Geometry: see drawing. Coordinates: mm, zero at the bounding-box minimum. A direction names the side the tool comes from. Coordinates: 2 decimals unless noted, no trailing zeros. Order: outer loops, then holes, each group sorted by start corner. A loop starts at its lowest first (then second) coordinate and runs counter-clockwise, first axis right, second up.
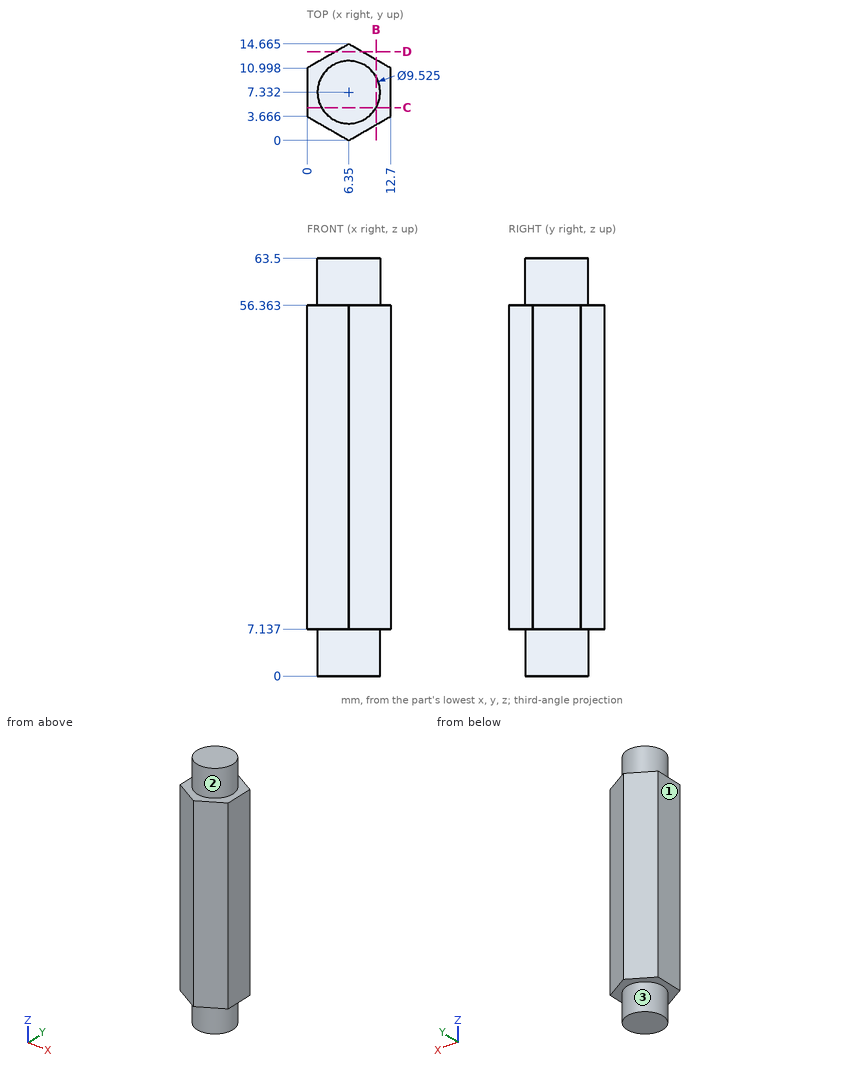
Item 1: Access query for the marked faces 1, 2 and 3. Directions: +Z, -Z, +X, -X, +Y, -Y. A direction counts if a zero-diameter tool reaches every point of the face in a straight line with its end or side. Return the directions, or none.
Response values:
face 1: +Z, -Z, -X, +Y, -Y
face 2: +Z
face 3: -Z
Item 2: Cut plane B-B on x = 10.5. Return loops of the section in (y, z) (1 decimal), then the cut area to 3 significant figures.
Response values:
outline: (2.4, 7.1) - (5, 7.1) - (5, 0) - (9.7, 0) - (9.7, 7.1) - (12.3, 7.1) - (12.3, 56.4) - (9.7, 56.4) - (9.7, 63.5) - (5, 63.5) - (5, 56.4) - (2.4, 56.4) - close
area: 553 mm2
Item 3: Pin query (flat end, axial travel): pin 1 Ø3 at (x, z) = (8.5, 21.5) entering from +Y; pin 2 Ø3 at (x, z) = (10, 20) entering from +Y; pin 3 Ø1.5 at (x, y) = (7.5, 13) entering from +Z. Return the tip coordinate at first contact, or that it passes through.
Response values:
pin 1: stops at y = 14.29
pin 2: stops at y = 13.42
pin 3: stops at z = 56.36
Item 4: Cut plane D-D on y = 13.5. Return loops of the section in (x, z).
Response values:
outline: (4.33, 7.14) - (8.37, 7.14) - (8.37, 56.36) - (4.33, 56.36) - close
Item 5: Cut plane C-C on y = 5. Return loops of the section in (x, z).
Response values:
outline: (0, 7.14) - (2.2, 7.14) - (2.2, 0) - (10.5, 0) - (10.5, 7.14) - (12.7, 7.14) - (12.7, 56.36) - (10.5, 56.36) - (10.5, 63.5) - (2.2, 63.5) - (2.2, 56.36) - (0, 56.36) - close
Item 6: Ray query, probe 1 along X at (y, z) = (2.75, 37) (1 decimal); probe 2 along Z at (x, y) = (12, 4.5); probe 3 along Y at (x, z) = (12, 26). Return the intervals inside material, ascending.
Response values:
probe 1: x = 1.6 to 11.1
probe 2: z = 7.14 to 56.36
probe 3: y = 3.26 to 11.4
